For this review, take the finished solid that the model builds, in its own axes (mm). A direction names the side the tool comes from. Round coordinates to 2 decimals unless told otherwise and drop trailing zeros. Use a Markdown table: item, result. Add a question column.
1) Clearance check with flat-ended pins moving along their axes: P1, Ø3, axis at y = 7, z = -16.5, coming from the -X side; P2, Ø1, axis at y = -24.5, z = -39.5, coming from the +X side; P3, Ø5, axis at y = -25.5, z = -70.5, coming from the +X side. State where each tip first meets the part, or that it passes through.
2) Draft analysis for pull direction Z (two halves, no side actions). For faces 1 (the face through (134.655, 0.814, -49.013)), 2 (the face through (-24.24, -6.11, -28.04)), 3 (the face through (152.4, 8, -56)), state which applies: pulls with the +Z half, pulls with the -Z half, needs draft (parallel to the pull), parting line crosses it, or undercut.
3) Wall thickness on line 1 along Z through (x, y) = (145, 0); line 2 along Z through (x, y) = (143.5, 0); line 3 along Y through (x, z) = (71, -46.5): over which ranges is each line inside the solid? List them lowest first. Write a range as [from, to].
4) Machinability: for faces 4 (the face through (145.961, 2.202, -57.366)), 5 (the face through (63, 29, -85)), which of the approach directions +Z, -Z, +X, -X, +Y, -Y give a long, thin tool a straight path to every point of the face, cutting with its end or side? Answer none if there is none.
```python
from build123d import *

# Parameters (mm, degrees)
F4_D     = 20.32
F4_DEPTH = 12.7
F4_TIP   = 6.1047438893
F3_R     = 5.08
F5_R     = 5.08


with BuildPart() as f1:
    # F0 (on Front) → F1 (revolve)
    with BuildSketch(Plane.XZ):
        Polygon((127, 0), (0, 0), (-25.4, -28.3980633142), (-25.4, -47.4480633142), (152.4, -47.4480633142), (152.4, -28.3980633142), align=None)
    revolve(axis=Axis((63.5, 0, -47.4480633142), (1, 0, 0)))

    # F4
    with Locations(Plane.YZ.offset(152.4)):
        with Locations((0, -47.4480633142)):
            Hole(F4_D / 2, depth=F4_DEPTH)
            with Locations((0, 0, -(F4_DEPTH + F4_TIP / 2))):  # 118° drill point
                Cone(0, F4_D / 2, F4_TIP, mode=Mode.SUBTRACT)

    # F3
    f3_edges = [f1.edges().sort_by_distance(p)[0] for p in [
        (127, 0, -94.896127),
    ]]
    fillet(f3_edges, radius=F3_R)

    # F5
    f5_edges = [f1.edges().sort_by_distance(p)[0] for p in [
        (0, 0, -94.896127),
    ]]
    fillet(f5_edges, radius=F5_R)


solid = f1.part
```
Results list:
| question | item | result |
|---|---|---|
| 1 | P1 | x = -15.4 |
| 1 | P2 | x = 146.85 |
| 1 | P3 | x = 140.93 |
| 2 | face 1 | undercut |
| 2 | face 2 | parting line crosses it |
| 2 | face 3 | needs draft |
| 3 | line 1 | [-74.77, -57.61], [-37.29, -20.12] |
| 3 | line 2 | [-76.45, -57.61], [-37.29, -18.45] |
| 3 | line 3 | [-47.44, 47.44] |
| 4 | face 4 | +X |
| 4 | face 5 | +X, -X |
